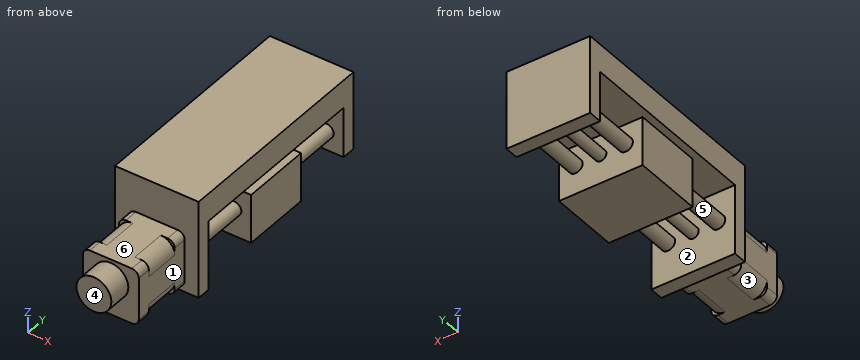
```python
from build123d import *

# Parameters (mm, degrees)
SKETCH1_W           = 60
SKETCH1_H           = 70
BOSS_EXTRUDE1_DEPTH = 10
SKETCH2_R           = 5
BOSS_EXTRUDE2_DEPTH = 135
SKETCH3_W           = 60
SKETCH3_H           = 70
BOSS_EXTRUDE3_DEPTH = 10
SKETCH4_R           = 4
BOSS_EXTRUDE4_DEPTH = 135
SKETCH6_W           = 60
SKETCH6_H           = 20
BOSS_EXTRUDE5_DEPTH = 135
SKETCH7_W           = 40
SKETCH7_H           = 40
BOSS_EXTRUDE6_DEPTH = 46
SKETCH8_R           = 12.5
BOSS_EXTRUDE7_DEPTH = 17
FILLET1_START       = -36
FILLET1_DEPTH       = 26
FILLET2_R           = 5
FILLET3_START       = -36
FILLET3_DEPTH       = 26
FILLET4_R           = 5
SKETCH9_W           = 60
SKETCH9_H           = 35
BOSS_EXTRUDE8_DEPTH = 50
SKETCH10_W          = 60
SKETCH10_H          = 10
CUT_EXTRUDE1_DEPTH  = 14


with BuildPart() as part:
    # Sketch1 → Boss-Extrude1 (new body)
    with BuildSketch(Plane(origin=(0, 0, 0), x_dir=(1, 0, 0), z_dir=(0, 1, 0))):
        Rectangle(SKETCH1_W, SKETCH1_H)
    extrude(amount=BOSS_EXTRUDE1_DEPTH)

    # Sketch2 → Boss-Extrude2 (add)
    with BuildSketch(Plane(origin=(0, 10, 0), x_dir=(1, 0, 0), z_dir=(0, 1, 0))):
        with Locations(Location((-18, 7, 0), (0, 0, 270))):
            Circle(SKETCH2_R)
        with Locations(Location((18, 7, 0), (0, 0, 270))):
            Circle(SKETCH2_R)
    extrude(amount=BOSS_EXTRUDE2_DEPTH)

    # Sketch3 → Boss-Extrude3 (add)
    with BuildSketch(Plane(origin=(0, 145, 0), x_dir=(1, 0, 0), z_dir=(0, 1, 0))):
        Rectangle(SKETCH3_W, SKETCH3_H)
    extrude(amount=BOSS_EXTRUDE3_DEPTH)

    # Sketch4 → Boss-Extrude4 (add)
    with BuildSketch(Plane(origin=(0, 10, 0), x_dir=(1, 0, 0), z_dir=(0, 1, 0))):
        with Locations(Location((0, 7, 0), (0, 0, 270))):
            Circle(SKETCH4_R)
    extrude(amount=BOSS_EXTRUDE4_DEPTH)

    # Sketch6 → Boss-Extrude5 (add)
    with BuildSketch(Plane(origin=(0, 10, 0), x_dir=(1, 0, 0), z_dir=(0, 1, 0))):
        with Locations((0, -25)):
            Rectangle(SKETCH6_W, SKETCH6_H)
    extrude(amount=BOSS_EXTRUDE5_DEPTH)

    # Sketch7 → Boss-Extrude6 (add)
    with BuildSketch(Plane.XZ):
        with Locations((0, -12)):
            Rectangle(SKETCH7_W, SKETCH7_H)
    extrude(amount=BOSS_EXTRUDE6_DEPTH)

    # Sketch8 → Boss-Extrude7 (add)
    with BuildSketch(Plane.XZ.offset(46)):
        with Locations(Location((0, -7, 0), (0, 0, 270))):
            Circle(SKETCH8_R)
    extrude(amount=BOSS_EXTRUDE7_DEPTH)

    # Fillet1: read off the stored shape, not the designer's step
    # Fillet1 outline → Fillet1 (cut)
    with BuildSketch(Plane(origin=(0, 0, 0), x_dir=(1, 0, 0), z_dir=(0, 1, 0)).offset(FILLET1_START)):
        with BuildLine():
            Line((-20, 32), (-20, 22))
            ThreePointArc((-20, 22), (-17.071067812, 29.071067812), (-10, 32))
            Line((-10, 32), (-20, 32))
        make_face()
    extrude(amount=FILLET1_DEPTH, mode=Mode.SUBTRACT)

    # Fillet2
    fillet2_edges = [part.edges().sort_by_distance(p)[0] for p in [
        (-20, -41, -32),
        (-20, -5, -32),
    ]]
    fillet(fillet2_edges, radius=FILLET2_R)

    # Fillet3: read off the stored shape, not the designer's step
    # Fillet3 outline → Fillet3 (cut)
    with BuildSketch(Plane(origin=(0, 0, 0), x_dir=(1, 0, 0), z_dir=(0, 1, 0)).offset(FILLET3_START)):
        with BuildLine():
            ThreePointArc((10, 32), (17.071067812, 29.071067812), (20, 22))
            Line((20, 22), (20, 32))
            Line((20, 32), (10, 32))
        make_face()
        with BuildLine():
            ThreePointArc((20, 2), (17.071067812, -5.071067812), (10, -8))
            Line((10, -8), (20, -8))
            Line((20, -8), (20, 2))
        make_face()
        with BuildLine():
            ThreePointArc((-10, -8), (-17.071067812, -5.071067812), (-20, 2))
            Line((-20, 2), (-20, -8))
            Line((-20, -8), (-10, -8))
        make_face()
    extrude(amount=FILLET3_DEPTH, mode=Mode.SUBTRACT)

    # Fillet4
    fillet4_edges = [part.edges().sort_by_distance(p)[0] for p in [
        (20, -41, -32),
        (20, -41, 8),
        (-20, -41, 8),
        (20, -5, 8),
        (20, -5, -32),
        (-20, -5, 8),
    ]]
    fillet(fillet4_edges, radius=FILLET4_R)

    # Sketch9 → Boss-Extrude8 (add)
    with BuildSketch(Plane(origin=(0, 52.5, 0), x_dir=(1, 0, 0), z_dir=(0, 1, 0))):
        with Locations((0, 9.5)):
            Rectangle(SKETCH9_W, SKETCH9_H)
    extrude(amount=BOSS_EXTRUDE8_DEPTH)

    # Sketch10 → Cut-Extrude1 (cut)
    with BuildSketch(Plane(origin=(0, 0, -35), x_dir=(-1, 0, 0), z_dir=(0, 0, -1))):
        with Locations((0, 150)):
            Rectangle(SKETCH10_W, SKETCH10_H)
    extrude(amount=-CUT_EXTRUDE1_DEPTH, mode=Mode.SUBTRACT)


solid = part.part
```
The listing builds one solid part. Answer for the finished solid, in the listing's coordinates (mm). Face numbers are marked on the shaded views. A direction names the side the tool comes from. Coordinates: 2 decimals unless noted, no trailing zeros. Write each loop counter-clockwise with the first axis right and the second up, starting at its lowest first coordinate (ties: lowest second). Pieces come first, ordered by that corner, then holes. Notation, with made-up numbers: (64, 86) -> (115, 86) arc R9 cw to (115, 101) -> close; hole circle Ø8 at (10.25, 84.25). An arc over 180 degrees is marked (long way). Write each question's results on one line, items separated by ' | '. Start each with the question number.
1) A tool of negligible diameter and unlimited length cuts with its end or side. For the marked faces 1, 2 and 3, from which of +Z, -Z, +X, -X, +Y, -Y can it reach the whole face along a straight path? Write none if from no direction.
2) A cutting plane is placed at B-B (z = -17). Determine the outline of the cut face in (x, y), then the cut area to 4 significant figures.
3) A cutting plane is placed at C-C (x = 0). Determine the outline of the cut face in (y, z), then the cut area to 4 significant figures.
4) Flat-ended cylindrical pins translate along their axes: pin 1 Ø6 at (x, y) = (-10, -19) entering from +Z; pin 2 Ø6 at (x, y) = (-1, 100) entering from -Z; pin 3 Ø8 at (x, z) = (12.5, -27) entering from +Y. Find the tip coordinate at first contact, or state that the pin passes through.
5) Straight lines are drawn through the part: probe 1 along Y at (x, z) = (-1, 7); probe 2 along Y at (x, z) = (3, -18.5); probe 3 along Y at (x, z) = (10, 9). For each, find the intervals that lie inside material, in ascending order.
6) A cutting plane is placed at A-A (y = 112). Determine the outline of the cut face in (x, z).
7) A cutting plane is placed at D-D (z = -7). Count the separate pieces of the cut face and the enclosed holes in it, then the cut area to 4 significant figures.
8) For a pull along Y with two mould halves and no side action, classify the marked faces 4, 5 and 6 as +Y half, -Y half, draft (parallel to the pull), parting line (faces both ways), or undercut.
Values follow:
1) face 1: +Z, -Z, +X, -Y | face 2: none | face 3: -Z, -X
2) outline: (-30, 0) -> (-20, 0) -> (-20, -46) -> (-7.5, -46) -> (-7.5, -63) -> (7.5, -63) -> (7.5, -46) -> (20, -46) -> (20, 0) -> (30, 0) -> (30, 10) -> (-30, 10) -> close; (-30, 52.5) -> (30, 52.5) -> (30, 102.5) -> (-30, 102.5) -> close; (-30, 145) -> (30, 145) -> (30, 155) -> (-30, 155) -> close | area: 6,295 mm²
3) outline: (-63, -19.5) -> (-46, -19.5) -> (-46, -32) -> (0, -32) -> (0, -35) -> (10, -35) -> (10, -11) -> (52.5, -11) -> (52.5, -27) -> (102.5, -27) -> (102.5, -11) -> (145, -11) -> (145, -21) -> (155, -21) -> (155, 35) -> (0, 35) -> (0, 8) -> (-46, 8) -> (-46, 5.5) -> (-63, 5.5) -> close; hole (10, -3) -> (52.5, -3) -> (52.5, 8) -> (102.5, 8) -> (102.5, -3) -> (145, -3) -> (145, 15) -> (10, 15) -> close | area: 8,655 mm²
4) pin 1: z = 8 | pin 2: z = -27 | pin 3: y = 102.5
5) probe 1: -46 to 10, 52.5 to 102.5, 145 to 155 | probe 2: -63 to 10, 52.5 to 102.5, 145 to 155 | probe 3: 0 to 10, 145 to 155
6) outline: (-30, 15) -> (30, 15) -> (30, 35) -> (-30, 35) -> close; circle Ø10 at (-18, -7); circle Ø8 at (0, -7); circle Ø10 at (18, -7)
7) separate pieces: 1 | enclosed holes: 4 | area: 8,845 mm²
8) face 4: -Y half | face 5: undercut | face 6: draft
